from build123d import *

# Parameters (mm, degrees)
SKETCH_1_W         = 37
SKETCH_1_H         = 30
EXTRUDE_1_DEPTH    = 34
SKETCH_2_R         = 12
EXTRUDE_2_DEPTH    = 6
SKETCH_3_R         = 14.5
EXTRUDE_3_DEPTH    = 26
SKETCH_4_R         = 20
EXTRUDE_4_DEPTH    = 2
DOME_1_FACE_RADIUS = 20
DOME_1_HEIGHT      = 4


with BuildPart() as part:
    # 草图1 → 凸台-拉伸1 (new body)
    with BuildSketch(Plane(origin=(0, 0, 0), x_dir=(1, 0, 0), z_dir=(0, 1, 0))):
        Rectangle(SKETCH_1_W, SKETCH_1_H)
    extrude(amount=EXTRUDE_1_DEPTH)

    # 草图2 → 凸台-拉伸2 (add)
    with BuildSketch(Plane(origin=(0, 34, 0), x_dir=(1, 0, 0), z_dir=(0, 1, 0))):
        with Locations(Location((0, 0, 0), (0, 0, 90))):
            Circle(SKETCH_2_R)
    extrude(amount=EXTRUDE_2_DEPTH)

    # 草图3 → 凸台-拉伸3 (add)
    with BuildSketch(Plane(origin=(0, 40, 0), x_dir=(1, 0, 0), z_dir=(0, 1, 0))):
        with Locations(Location((0, 0, 0), (0, 0, 90))):
            Circle(SKETCH_3_R)
    extrude(amount=EXTRUDE_3_DEPTH)

    # 草图4 → 凸台-拉伸4 (add)
    with BuildSketch(Plane(origin=(0, 66, 0), x_dir=(1, 0, 0), z_dir=(0, 1, 0))):
        with Locations(Location((0, 0, 0), (0, 0, 270))):
            Circle(SKETCH_4_R)
    extrude(amount=EXTRUDE_4_DEPTH)

    # 圆顶1: a dome of height H over a round flat face of radius A is a cap of a sphere of radius (A * A + H * H) / (2 * H)
    dome_1_r = (DOME_1_FACE_RADIUS * DOME_1_FACE_RADIUS + DOME_1_HEIGHT * DOME_1_HEIGHT) / (2 * DOME_1_HEIGHT)
    dome_1_base = Plane((0, 68, 0), z_dir=(0, 1, 0))
    with Locations(dome_1_base.offset(DOME_1_HEIGHT - dome_1_r)):
        dome_1_ball = Sphere(dome_1_r, mode=Mode.PRIVATE)
    add(split(dome_1_ball, bisect_by=dome_1_base, keep=Keep.TOP, mode=Mode.PRIVATE))


solid = part.part
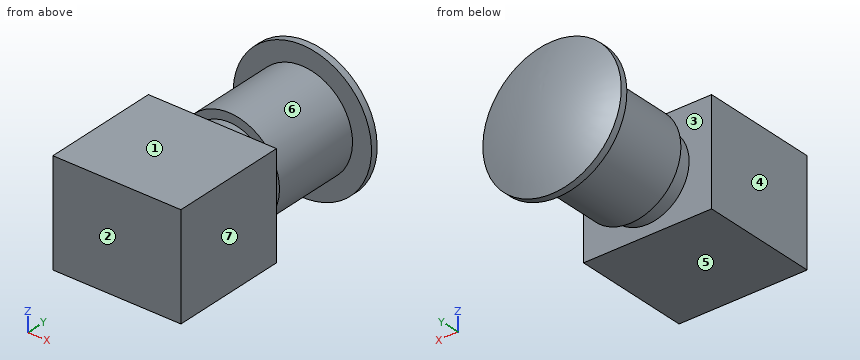
Model file for the job. Use its own axes, mm. Face numbers are marked on the shaded views. A direction names the side the tool comes from. Give positions to 0.01 mm unless a question says otherwise; leave off trailing zeros. Loops run counter-clockwise (first coordinate to the right, second up) from the corner with the lowest first, then second, coordinate; pieces in that order, holes last.
Item 1: Slice it at C-C (x = 0). Write the cut outline in (y, z), plus the area to 3 significant figures.
Check values:
outline: (0, -15) - (34, -15) - (34, -12) - (40, -12) - (40, -14.5) - (66, -14.5) - (66, -20) - (68, -20) arc R52 ccw to (68, 20) - (66, 20) - (66, 14.5) - (40, 14.5) - (40, 12) - (34, 12) - (34, 15) - (0, 15) - close
area: 2,110 mm2
Item 2: Slice it at B-B (x = -13). Write the cut outline in (y, z), plus the area to 3 significant figures.
Check values:
outline: (0, -15) - (34, -15) - (34, 15) - (0, 15) - close; (40, -6.42) - (66, -6.42) - (66, -15.2) - (68, -15.2) arc R50.35 ccw to (68, 15.2) - (66, 15.2) - (66, 6.42) - (40, 6.42) - close
area: 1,460 mm2
Item 3: Slice it at D-D (y = 49). Write the cut outline in (x, z).
Check values:
outline: circle Ø29 at (0, 0)
Item 4: Drop flat-ended pins along their axis: P1, Ø1.5, axis at y = 10, z = -2, coming from the -X side; P2, Ø3, axis at y = 12.5, z = 4.5, coming from the +X side; P3, Ø20, axis at x = 6.5, z = -5.5, coming from the -Y side; P4, Ø6, axis at y = 49, z = 15, coming from the +X side. Give the stop position or say it passes through.
Check values:
P1: stops at x = -18.5
P2: stops at x = 18.5
P3: stops at y = 0
P4: stops at x = 8.14
Item 5: Drill centre lines: line 1 along X through (y, z) = (12.5, -1); line 2 along Z through (x, y) = (-11, 11.5); line 3 along Y through (x, z) = (-16, -3). Where is each one in solid material? Low to high.
Check values:
line 1: x = -18.5 to 18.5
line 2: z = -15 to 15
line 3: y = 0 to 34, 66 to 69.39
Item 6: Mould opens along Y. For the marked faces 1, 2 and 3 say: +Y half, -Y half, draft (parallel to the pull), parting line (faces both ways), or undercut.
Check values:
face 1: draft
face 2: -Y half
face 3: undercut
Item 7: Which spindle directions (+Z, -Z, +X, -X, +Y, -Y) get a long thin tool onto all of the face, cutting with end or side? Do the marked faces 4, 5, 6 and 7. Say none if no direction does.
Check values:
face 4: +Z, -Z, -X, -Y
face 5: -Z, +X, -X, -Y
face 6: none
face 7: +Z, -Z, +X, -Y
Item 8: Slice it at A-A (z = 0). Write the cut outline in (x, y).
Check values:
outline: (-20, 66) - (-14.5, 66) - (-14.5, 40) - (-12, 40) - (-12, 34) - (-18.5, 34) - (-18.5, 0) - (18.5, 0) - (18.5, 34) - (12, 34) - (12, 40) - (14.5, 40) - (14.5, 66) - (20, 66) - (20, 68) arc R52 ccw to (-20, 68) - close
